from build123d import *

# Parameters (mm, degrees)
BOSS_EXTRUDE1_DEPTH = 1.5
SKETCH2_W           = 35.686807758
SKETCH2_H           = 1.5
BOSS_EXTRUDE2_DEPTH = 1.5
SKETCH3_W           = 11.9
SKETCH3_H           = 1.5
BOSS_EXTRUDE3_DEPTH = 1.5
SKETCH4_W           = 23.7
SKETCH4_H           = 1.5
BOSS_EXTRUDE4_DEPTH = 1.5
BOSS_EXTRUDE5_DEPTH = 3.55
SKETCH6_W           = 4.966668371
SKETCH6_H           = 1.5
SKETCH6_W_2         = 5.4
SKETCH6_H_2         = 1.85
BOSS_EXTRUDE6_DEPTH = 5


with BuildPart() as part:
    # Sketch1 → Boss-Extrude1 (new body)
    with BuildSketch(Plane(origin=(0, 0, 0), x_dir=(1, 0, 0), z_dir=(0, 1, 0))):
        Polygon((-75.339050621, 34.683913692), (-39.639050621, 34.683913692), (-39.639050621, 24.283913692), (-53.039050621, 24.283913692), (-53.289050621, 1.283913692), (-70.339050621, 1.283913692), (-70.339050621, 12.483913692), (-75.339050621, 12.483913692), (-75.339050621, 24.283913692), align=None)
    extrude(amount=BOSS_EXTRUDE1_DEPTH)

    # Sketch2 → Boss-Extrude2 (add)
    with BuildSketch(Plane(origin=(0, 0, -34.683913692), x_dir=(-1, 0, 0), z_dir=(0, 0, -1))):
        with Locations((57.4824545, 0.75)):
            Rectangle(SKETCH2_W, SKETCH2_H)
    extrude(amount=BOSS_EXTRUDE2_DEPTH)

    # Sketch3 → Boss-Extrude3 (add)
    with BuildSketch(Plane(origin=(-39.639050621, 0, 0), x_dir=(0, 0, -1), z_dir=(1, 0, 0))):
        with Locations((30.233913692, 0.75)):
            Rectangle(SKETCH3_W, SKETCH3_H)
    extrude(amount=BOSS_EXTRUDE3_DEPTH)

    # Sketch4 → Boss-Extrude4 (add)
    with BuildSketch(Plane.ZY.offset(75.325858379)):
        with Locations((-24.333913692, 0.75)):
            Rectangle(SKETCH4_W, SKETCH4_H)
    extrude(amount=BOSS_EXTRUDE4_DEPTH)

    # Sketch5 → Boss-Extrude5 (add)
    with BuildSketch(Plane(origin=(0, 1.5, 0), x_dir=(1, 0, 0), z_dir=(0, 1, 0))):
        Polygon((-75.525858379, 34.683913692), (-75.525858379, 30.004194868), (-76.825858379, 30.004194868), (-76.825858379, 36.183913692), (-70.559190008, 36.183913692), (-70.559190008, 34.683913692), align=None)
        Polygon((-39.439050621, 34.683913692), (-39.439050621, 29.683913692), (-38.139050621, 29.683913692), (-38.139050621, 36.183913692), (-44.839050621, 36.183913692), (-44.839050621, 34.683913692), align=None)
    extrude(amount=BOSS_EXTRUDE5_DEPTH)

    # Sketch6 → Boss-Extrude6 (add)
    with BuildSketch(Plane.XY.offset(-34.683913692)):
        with Locations((-73.042524194, 4.3)):
            Rectangle(SKETCH6_W, SKETCH6_H)
        with Locations((-42.139050621, 4.125)):
            Rectangle(SKETCH6_W_2, SKETCH6_H_2)
    extrude(amount=BOSS_EXTRUDE6_DEPTH)


solid = part.part
Design review of the part built by this model. Coordinates are the model's own, in mm. A direction names the side the tool comes from. Coordinates: 2 decimals unless noted, no trailing zeros. Loops run counter-clockwise (first coordinate to the right, second up) from the corner with the lowest first, then second, coordinate; pieces in that order, holes last. Notation, with made-up numbers: M 76.25,72 L 132.25,72 A29 cw 132.25,110 Z; hole C 49.25,73.25 d6. An arc over 180 degrees is marked long. Use one line per item in the form item = value.
(1) Consider section A-A (y = 2). Write out the cut boundary in (x, z).
Return value:
outline = M -76.83,-36.18 L -70.56,-36.18 L -70.56,-34.68 L -75.53,-34.68 L -75.53,-30 L -76.83,-30 Z; M -44.84,-36.18 L -38.14,-36.18 L -38.14,-29.68 L -39.44,-29.68 L -39.44,-34.68 L -44.84,-34.68 Z
(2) Draft analysis for pull direction Y (two halves, no side actions). For faces 1 (the face through (-75.526, 3, -32)), 2 (the face through (-62, 1, -1.284)), 3 (the face through (-74, 5.05, -33)), 4 (the face through (-62, 0, -23)), state which applies: pulls with the +Y half, pulls with the -Y half, needs draft (parallel to the pull), parting line crosses it, or undercut.
Return value:
face_1 = undercut
face_2 = needs draft
face_3 = pulls with the +Y half
face_4 = pulls with the -Y half
(3) Consider section C-C (y = 4.5). Write out the cut boundary in (x, z).
Return value:
outline = M -76.83,-36.18 L -70.56,-36.18 L -70.56,-29.68 L -75.53,-29.68 L -75.53,-30 L -76.83,-30 Z; M -44.84,-36.18 L -38.14,-36.18 L -38.14,-29.68 L -44.84,-29.68 Z
(4) Consider section D-D (z = -25.5). Write out the cut boundary in (x, y), and give its area (3 significant figures).
Return value:
outline = M -76.83,0 L -38.14,0 L -38.14,1.5 L -76.83,1.5 Z
area = 58.0 mm2
(5) Consider section B-B (x = -40.5). Write out the cut boundary in (y, z).
Return value:
outline = M 0,-36.18 L 5.05,-36.18 L 5.05,-29.68 L 3.2,-29.68 L 3.2,-34.68 L 1.5,-34.68 L 1.5,-24.28 L 0,-24.28 Z
(6) For line 1 along Y through (x, z) = (-53.5, -33); line 2 along Z through (x, y) = (-72.5, 0.45); line 3 along Z through (x, y) = (-41.5, 4.6), list the stretches that pass through material, from the lowest coordinate up. Write a range as from..to.
Return value:
line_1 = 0..1.5
line_2 = -36.18..-12.48
line_3 = -36.18..-29.68
(7) Clearance check with flat-ended pins moving along their axes: P1, Ø10, axis at x = -58.5, z = -7.5, coming from the +Y side; P2, Ø2.5, axis at x = -72, y = 3, coming from the +Z side; P3, Ø0.5, axis at x = -42.5, y = 2.5, coming from the +Z side. State where each tip first meets the part, or that it passes through.
Return value:
P1 = 1.5
P2 = -29.68
P3 = -34.68
(8) For faces 5 (the face through (-41, 4, -29.684)), 6 (the face through (-76.826, 1, -27)), 7 (the face through (-73, 3, -34.684)), 8 (the face through (-70.559, 4, -34)), 9 (the face through (-74, 1, -12.484)), list the 3-axis set-ups (+Z, -Z, +X, -X, +Y, -Y) from which the entire face can be reached by the end or side of a thin tool; tool diameter is ignored.
Return value:
face_5 = +Z, +X, -X, +Y
face_6 = +Z, -Z, -X, +Y, -Y
face_7 = +Z
face_8 = +Z, -Z, +Y
face_9 = +Z, -X, +Y, -Y
